from build123d import *

# Parameters (mm, degrees)
BOSS_EXTRUDE1_DEPTH = 10
SKETCH4_W           = 40.2
SKETCH4_H           = 9.2
CUT_EXTRUDE1_DEPTH  = 49.176757882
SKETCH3_R           = 2.1
CUT_EXTRUDE2_DEPTH  = 2.4
SKETCH5_R           = 1.6
CUT_EXTRUDE3_DEPTH  = 2.4
FILLET1_R           = 1


with BuildPart() as part:
    # Sketch1 → Boss-Extrude1 (new body)
    with BuildSketch(Plane(origin=(0, 0, 0), x_dir=(0, 0, -1), z_dir=(1, 0, 0))):
        Polygon((0, 11.6), (0, 0), (45, 0), (45, 14), (0, 14), (-27, 14), (-27, 11.6), align=None)
    extrude(amount=BOSS_EXTRUDE1_DEPTH)

    # Sketch4 → Cut-Extrude1 (cut, through all)
    with BuildSketch(Plane(origin=(10, 0, 0), x_dir=(0, 0, -1), z_dir=(1, 0, 0))):
        with Locations((22.5, 7)):
            Rectangle(SKETCH4_W, SKETCH4_H)
    extrude(amount=-CUT_EXTRUDE1_DEPTH, mode=Mode.SUBTRACT)

    # Sketch3 → Cut-Extrude2 (cut)
    with BuildSketch(Plane(origin=(0, 0, 0), x_dir=(1, 0, 0), z_dir=(0, 1, 0))):
        with Locations(Location((5, 32.5, 0), (0, 0, 90))):
            Circle(SKETCH3_R)
        with Locations(Location((5, 12.5, 0), (0, 0, 90))):
            Circle(SKETCH3_R)
    extrude(amount=CUT_EXTRUDE2_DEPTH, mode=Mode.SUBTRACT)

    # Sketch5 → Cut-Extrude3 (cut)
    with BuildSketch(Plane(origin=(0, 14, 0), x_dir=(1, 0, 0), z_dir=(0, 1, 0))):
        with Locations(Location((5, 23, 0), (0, 0, 270))):
            Circle(SKETCH5_R)
        with Locations(Location((5, -22, 0), (0, 0, 270))):
            Circle(SKETCH5_R)
    extrude(amount=-CUT_EXTRUDE3_DEPTH, mode=Mode.SUBTRACT)

    # Fillet1
    fillet1_edges = [part.edges().sort_by_distance(p)[0] for p in [
        (5, 0, 0),
        (5, 11.6, 0),
        (5, 11.6, 27),
        (5, 14, 27),
        (5, 14, -45),
        (5, 0, -45),
        (5, 2.4, -2.4),
        (5, 11.6, -2.4),
        (5, 11.6, -42.6),
        (5, 2.4, -42.6),
    ]]
    fillet(fillet1_edges, radius=FILLET1_R)


solid = part.part
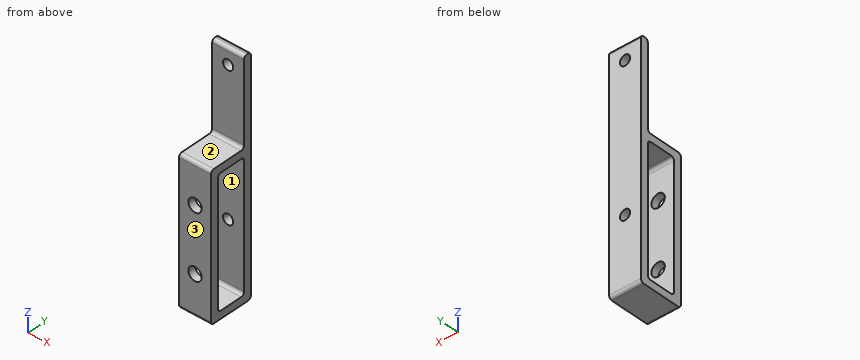
For this review, take the finished solid that the model builds, in its own axes (mm). Face numbers are marked on the shaded views. A direction names the side the tool comes from. Give positions to 0.01 mm unless a question says otherwise; leave off trailing zeros. Loops run counter-clockwise (first coordinate to the right, second up) from the corner with the lowest first, then second, coordinate; pieces in that order, holes last.
Item 1: Take a section at D-D, the plane z = -32.5. State the section outline as (x, y) points, and give its area (3 significant figures).
Item 2: For line 1 along X through (y, z) = (0.9, -12.5); line 2 along Y through (x, z) = (4.5, -41); line 3 along Z through (x, y) = (7.5, 8.5), list the stretches that pass through material, from the lowest coordinate up.
Item 3: Take a section at C-C, the plane z = 22. State the section outline as (x, y) points.
Item 4: Insertion check: pin 1 (6 mm diameter, centred on y = 10, z = -24.5, fed in from -X); pin 2 (2.5 mm diameter, centred on x = 5, z = -12.5, fed in from -Y); pin 3 (3.5 mm diameter, centred on x = 3, y = 8.5, fed in from +Z); pin 4 (3 mm diameter, centred on x = 5, z = -23, fed in from +Y). Each pin has a flat end and moves straight along its axis. Give the tip position at first contact, or say it passes through.
Item 5: Take a section at B-B, the plane x = 1.25. State the section outline as (y, z) points.
Item 6: Tool access review of the marked faces 1, 2 and 3: name each direction out of +Z, -Z, +X, -X, +Y, -Y from which nothing blocks a thin tool from reaching the whole face with its end or side.
Item 7: Take a section at A-A, the plane z = -23. State the section outline as (x, y) points.
Calculated:
1. outline: (0, 0) - (2.9, 0) - (2.9, 2.4) - (0, 2.4) - close; (0, 11.6) - (10, 11.6) - (10, 14) - (0, 14) - close; (7.1, 0) - (10, 0) - (10, 2.4) - (7.1, 2.4) - close
1. area: 37.9 mm2
2. line 1: x = 0 to 2.9, 7.1 to 10
2. line 2: y = 0 to 2.4, 11.6 to 14
2. line 3: z = -45 to -42.6, -2.4 to 0
3. outline: (0, 11.6) - (3.4, 11.6) - (3.4, 14) - (0, 14) - close; (6.6, 11.6) - (10, 11.6) - (10, 14) - (6.6, 14) - close
4. pin 1: stops at x = 0
4. pin 2: stops at y = 11.6
4. pin 3: stops at z = 0
4. pin 4: stops at y = 2.4
5. outline: (0, -44) arc R1 ccw to (1, -45) - (13, -45) arc R1 ccw to (14, -44) - (14, 26) arc R1 ccw to (13, 27) - (12.6, 27) arc R1 ccw to (11.6, 26) - (11.6, 1) arc R1 cw to (10.6, 0) - (1, 0) arc R1 ccw to (0, -1) - close; hole (2.4, -41.6) arc R1 ccw to (3.4, -42.6) - (10.6, -42.6) arc R1 ccw to (11.6, -41.6) - (11.6, -3.4) arc R1 ccw to (10.6, -2.4) - (3.4, -2.4) arc R1 ccw to (2.4, -3.4) - close
6. face 1: +X, -X
6. face 2: +Z, +X, -X, -Y
6. face 3: +Z, -Z, +X, -X, -Y
7. outline: (0, 0) - (10, 0) - (10, 2.4) - (0, 2.4) - close; (0, 11.6) - (3.4, 11.6) - (3.4, 14) - (0, 14) - close; (6.6, 11.6) - (10, 11.6) - (10, 14) - (6.6, 14) - close
